Autodesk Inventor part; units mm, degrees
ref_plane "YZ Plane" through (0, 0, 0) normal (1, 0, 0) x (0, 1, 0)
ref_plane "XZ Plane" through (0, 0, 0) normal (0, 1, 0) x (-1, 0, 0)
ref_plane "XY Plane" through (0, 0, 0) normal (0, 0, 1) x (1, 0, 0)
ref_plane "Work Plane3" through (0, 0, 0) normal (0, -1, 0) x (1, 0, 0)
sketch "Sketch2" plane through (0, 0, 0) normal (0, -1, 0) x (1, 0, 0)
  circle A0 centre (0, 0) radius 22.352
  arc A1 (22.352, 0) -> (-22.352, 0) centre (0, 0) ccw
  line L0 (22.352, 0) -> (-22.352, 0)
extrude "Extrusion2" add sketch "Sketch2" along normal blind 2
ref_plane "Work Plane5" through (0, 0, 0) normal (0, 1, 0) x (1, 0, 0)
sketch "Sketch3" plane through (0, 0, 0) normal (0, 1, 0) x (1, 0, 0)
  circle A0 centre (0, 0) radius 7
  line L0 (-20.955, 0) -> (20.955, 0)
  line L1 (-7, 0) -> (7, 0)
  dimension "d6" = 14
extrude "Extrusion3" add sketch "Sketch3" along normal blind 7.62
ref_plane "Work Plane4" through (0, -2, 0) normal (0, -1, 0) x (1, 0, 0)
sketch "Sketch4" plane through (0, -2, 0) normal (0, -1, 0) x (1, 0, 0)
  circle A0 centre (0, 0) radius 6
  dimension "d9" = 12
extrude "Extrusion4" cut sketch "Sketch4" against normal blind 8.5725
ref_plane "Work Plane6" through (0, 7.62, 0) normal (0, 1, 0) x (1, 0, 0)
sketch "Sketch5" plane through (0, 7.62, 0) normal (0, 1, 0) x (1, 0, 0)
  circle A0 centre (0, 0) radius 4
  line L0 (7, 0) -> (-7, 0)
  line L1 (4, 0) -> (-4, 0)
  dimension "d12" = 8
extrude "Extrusion5" add sketch "Sketch5" along normal blind 10.16
ref_plane "Work Plane7" through (0, 6.5725, 0) normal (0, -1, 0) x (1, 0, 0)
sketch "Sketch6" plane through (0, 6.5725, 0) normal (0, -1, 0) x (1, 0, 0)
  circle A0 centre (0, 0) radius 3
  dimension "d15" = 6
extrude "Extrusion6" cut sketch "Sketch6" against normal blind 10.16
ref_plane "Work Plane1" through (0, 25.4, 0) normal (0, 1, 0) x (1, 0, 0)
sketch "Sketch7" plane through (0, 25.4, 0) normal (0, 1, 0) x (1, 0, 0)
  point P0 (0, 0)
ref_plane "Work Plane2" through (0, 25.4, 0) normal (0, 1, 0) x (1, 0, 0)
sketch "Sketch12" plane through (0, 25.4, 0) normal (0, 1, 0) x (1, 0, 0)
  circle A0 centre (0, 0) radius 16.1182
  circle A1 centre (0, 0) radius 32.5204
extrude "Extrusion10" cut sketch "Sketch12" against normal up to surface (25.4 mm away)
properties part number "mold"
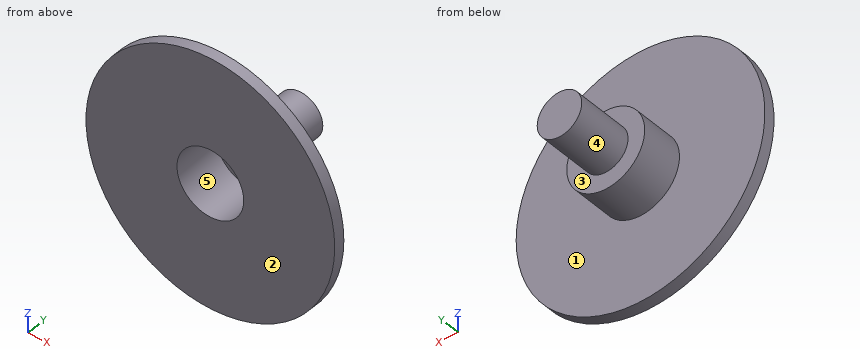
Input: part model. Units: mm. Frame: model coordinates. Face numbers are marked on the shaded views. A direction names the side the tool comes from. Coordinates: 2 decimals unless noted, no trailing zeros. Order: outer loops, then holes, each group sorted by start corner. A loop starts at its lowest first (then second) coordinate and runs counter-clockwise, first axis right, second up. Notation, with made-up numbers: (-11.75, 38) - (6.25, 38) arc R14 cw to (6.25, 47) - close; hole circle Ø6 at (-23.75, 69). An arc over 180 degrees is marked (long way). Put each result on its own line as item: value.
1. Cut plane B-B on z = 0. Return the cut outline in (x, y).
Report:
outline: (-22.35, -2) - (-6, -2) - (-6, 6.57) - (-3, 6.57) - (-3, 16.73) - (3, 16.73) - (3, 6.57) - (6, 6.57) - (6, -2) - (22.35, -2) - (22.35, 0) - (7, 0) - (7, 7.62) - (4, 7.62) - (4, 17.78) - (-4, 17.78) - (-4, 7.62) - (-7, 7.62) - (-7, 0) - (-22.35, 0) - close
2. Cut plane A-A on x = 0. Return the cut outline in (y, z), then the cut area to 3 significant figures.
Report:
outline: (-2, -22.35) - (0, -22.35) - (0, -7) - (7.62, -7) - (7.62, -4) - (17.78, -4) - (17.78, 4) - (7.62, 4) - (7.62, 7) - (0, 7) - (0, 22.35) - (-2, 22.35) - (-2, 6) - (6.57, 6) - (6.57, 3) - (16.73, 3) - (16.73, -3) - (6.57, -3) - (6.57, -6) - (-2, -6) - close
area: 114 mm2
3. Cut plane C-C on y = 4.5. Return the cut outline in (x, z).
Report:
outline: circle Ø14 at (0, 0); hole circle Ø12 at (0, 0)
4. Contact query for flat-ended pins moving along their axis: pin 1 Ø1 at (x, z) = (6, -10.5) entering from +Y; pin 2 Ø10 at (y, z) = (7.5, -7.5) entering from -X; pin 3 Ø4 at (y, z) = (13, 3) entering from +X; pin 4 Ø6 at (x, y) = (-17, 5) entering from -Z. Output: stop coordinate, or through.
Report:
pin 1: stops at y = 0
pin 2: stops at x = -6.54
pin 3: stops at x = 3.87
pin 4: passes through
5. Cut plane D-D on x = 11.5. Return the cut outline in (y, z), then the cut area to 3 significant figures.
Report:
outline: (-2, -19.17) - (0, -19.17) - (0, 19.17) - (-2, 19.17) - close
area: 76.7 mm2
6. Line query: line 1 along Z through (x, y) = (0, 14.25); line 2 along X through (y, z) = (2.75, -2.5); line 3 along Y through (x, z) = (-12, 0). Output: solid intervals per line, ascending.
Report:
line 1: z = -4 to -3, 3 to 4
line 2: x = -6.54 to -5.45, 5.45 to 6.54
line 3: y = -2 to 0
7. Draft query along Z for the marked faces 3, 4 and 5. Return one class per face: pulls with the +Z half, pulls with the -Z half, needs draft (parallel to the pull), parting line crosses it, or undercut.
Report:
face 3: needs draft
face 4: parting line crosses it
face 5: undercut
8. Reachability of the marked faces 1 and 2 from +Z, -Z, +X, -X, +Y, -Y: full face, straight path, thin tool, end or side. Return the list, or none.
Report:
face 1: +Y
face 2: +Z, -Z, +X, -X, -Y
